Here's how the part is built. I have some questions about the finished solid (model axes, mm). Face numbers are marked on the shaded views. Give positions to 0.01 mm unless a question says otherwise; leave off trailing zeros. Order: outer loops, then holes, each group sorted by start corner. A loop starts at its lowest first (then second) coordinate and runs counter-clockwise, first axis right, second up.
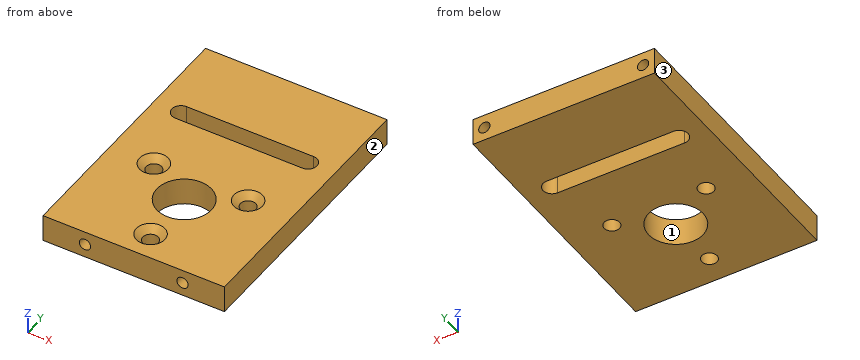
from build123d import *

# Parameters (mm, degrees)
SKETCH1_W                                           = 40
SKETCH1_H                                           = 58
BOSS_EXTRUDE1_DEPTH                                 = 3
SKETCH2_R                                           = 6
CUT_EXTRUDE1_DEPTH                                  = 36.73513677
CSK_FOR_M3_COUNTERSUNK_FLAT_HEAD_SCREW1_D           = 3.4
CSK_FOR_M3_COUNTERSUNK_FLAT_HEAD_SCREW1_CSINK_D     = 6.3
CSK_FOR_M3_COUNTERSUNK_FLAT_HEAD_SCREW1_CSINK_ANGLE = 90
TAP_DRILL_FOR_M3_TAP1_D                             = 2.5
TAP_DRILL_FOR_M3_TAP1_DEPTH                         = 9
TAP_DRILL_FOR_M3_TAP1_TIP                           = 0.751075774
TAP_DRILL_FOR_M3_TAP2_D                             = 2.5
TAP_DRILL_FOR_M3_TAP2_DEPTH                         = 9
TAP_DRILL_FOR_M3_TAP2_TIP                           = 0.751075774
CUT_EXTRUDE3_DEPTH                                  = 36.73513677


with BuildPart() as part:
    # Sketch1 → Boss-Extrude1 (new, symmetric)
    with BuildSketch(Plane.XY):
        Rectangle(SKETCH1_W, SKETCH1_H)
    extrude(amount=BOSS_EXTRUDE1_DEPTH, both=True)

    # Sketch2 → Cut-Extrude1 (cut, through all)
    with BuildSketch(Plane.XY.offset(3)):
        with Locations((0, -11)):
            Circle(SKETCH2_R)
    extrude(amount=-CUT_EXTRUDE1_DEPTH, mode=Mode.SUBTRACT)

    # CSK for M3 Countersunk Flat Head Screw1 (through all)
    with Locations(Plane.XY.offset(3)):
        with Locations((0, -23), (-10.392304845, -5), (10.392304845, -5)):
            CounterSinkHole(CSK_FOR_M3_COUNTERSUNK_FLAT_HEAD_SCREW1_D / 2, CSK_FOR_M3_COUNTERSUNK_FLAT_HEAD_SCREW1_CSINK_D / 2, counter_sink_angle=CSK_FOR_M3_COUNTERSUNK_FLAT_HEAD_SCREW1_CSINK_ANGLE)

    # Tap Drill for M3 Tap1
    with Locations(Plane(origin=(0, -29, 0), x_dir=(-1, 0, 0), z_dir=(0, -1, 0))):
        with Locations((10.75, 0), (-10.75, 0)):
            Hole(TAP_DRILL_FOR_M3_TAP1_D / 2, depth=TAP_DRILL_FOR_M3_TAP1_DEPTH)
            with Locations((0, 0, -(TAP_DRILL_FOR_M3_TAP1_DEPTH + TAP_DRILL_FOR_M3_TAP1_TIP / 2))):  # 118° drill point
                Cone(0, TAP_DRILL_FOR_M3_TAP1_D / 2, TAP_DRILL_FOR_M3_TAP1_TIP, mode=Mode.SUBTRACT)

    # Tap Drill for M3 Tap2
    with Locations(Plane(origin=(0, 29, 0), x_dir=(1, 0, 0), z_dir=(0, 1, 0))):
        with Locations((17.5, 0), (-17.5, 0)):
            Hole(TAP_DRILL_FOR_M3_TAP2_D / 2, depth=TAP_DRILL_FOR_M3_TAP2_DEPTH)
            with Locations((0, 0, -(TAP_DRILL_FOR_M3_TAP2_DEPTH + TAP_DRILL_FOR_M3_TAP2_TIP / 2))):  # 118° drill point
                Cone(0, TAP_DRILL_FOR_M3_TAP2_D / 2, TAP_DRILL_FOR_M3_TAP2_TIP, mode=Mode.SUBTRACT)

    # Sketch10 → Cut-Extrude3 (cut, through all)
    with BuildSketch(Plane.XY.offset(3)):
        with BuildLine():
            Line((-14, 12.5), (14, 12.5))
            ThreePointArc((14, 12.5), (16, 10.5), (14, 8.5))
            Line((14, 8.5), (-14, 8.5))
            ThreePointArc((-14, 8.5), (-16, 10.5), (-14, 12.5))
        make_face()
    extrude(amount=-CUT_EXTRUDE3_DEPTH, mode=Mode.SUBTRACT)


solid = part.part
Q1. If we section it at C-C on x = -4.5: List the corners of the cut face in (y, z) for me, plus the area to 3 significant figures.
Filled sheet:
outline: (-29, -3) - (-14.97, -3) - (-14.97, 3) - (-29, 3) - close; (-7.03, -3) - (8.5, -3) - (8.5, 3) - (-7.03, 3) - close; (12.5, -3) - (29, -3) - (29, 3) - (12.5, 3) - close
area: 276 mm2
Q2. I need wall thicknesses on L1, parallel to Y at x = -5, z = 0.1; L2, parallel to Y at x = 0.5, z = -1.55; L3, parallel to X at y = -6.5, z = -1.25. Which ranges of each line are inside material? Lowest first, please.
Filled sheet:
L1: y = -29 to -14.32, -7.68 to 8.5, 12.5 to 29
L2: y = -29 to -24.62, -21.38 to -16.98, -5.02 to 8.5, 12.5 to 29
L3: x = -20 to -11.19, -9.59 to -3.97, 3.97 to 9.59, 11.19 to 20
Q3. If we section it at B-B on y = -11: List the corners of the cut face in (x, z) for me.
Filled sheet:
outline: (-20, -3) - (-6, -3) - (-6, 3) - (-20, 3) - close; (6, -3) - (20, -3) - (20, 3) - (6, 3) - close
Q4. If we section it at A-A on x = 0: List the corners of the cut face in (y, z) for me, plus the area to 3 significant figures.
Filled sheet:
outline: (-29, -3) - (-24.7, -3) - (-24.7, 1.55) - (-26.15, 3) - (-29, 3) - close; (-21.3, -3) - (-17, -3) - (-17, 3) - (-19.85, 3) - (-21.3, 1.55) - close; (-5, -3) - (8.5, -3) - (8.5, 3) - (-5, 3) - close; (12.5, -3) - (29, -3) - (29, 3) - (12.5, 3) - close
area: 229 mm2
Q5. Thinking about a two-plate mould opening in X: for the marked faces 1, 2 and 3, which applies, released by +X, released by -X, zero draft, split by the parting line, or undercut?
Filled sheet:
face 1: undercut
face 2: released by +X
face 3: released by -X
Q6. If we section it at D-D on y = 10.5: List the corners of the cut face in (x, z) for me, plus the area to 3 significant figures.
Filled sheet:
outline: (-20, -3) - (-16, -3) - (-16, 3) - (-20, 3) - close; (16, -3) - (20, -3) - (20, 3) - (16, 3) - close
area: 48.0 mm2
Q7. I'm going to push flat-ended pins straight in: P1, Ø1.5, axis at x = -17.5, z = 0, coming from the +Y side; P2, Ø7, axis at x = 0, y = -11, coming from the -Z side. Where does each tip first touch, or does it pass through?
Filled sheet:
P1: stops at y = 19.7
P2: passes through
